For this review, take the finished solid that the model builds, in its own axes (mm). A direction names the side the tool comes from. Give positions to 0.01 mm unless a question says otherwise; leave off trailing zeros. Write each loop counter-clockwise with the first axis right and the second up, starting at its lowest first coordinate (ties: lowest second). Pieces come first, ordered by that corner, then holes. Notation, with made-up numbers: (76.5, -34) -> (108.5, -34) arc R17 cw to (108.5, -23) -> close; hole circle Ø7 at (13, -30.75). An arc over 180 degrees is marked (long way). Return JSON: item names as keys, results as strings.
from build123d import *

# Parameters (mm, degrees)
PAD_DEPTH    = 10
SKETCH001_R  = 2
POCKET_DEPTH = 31
CHAMFER_SIZE = 4
FILLET_R     = 4


with BuildPart() as part:
    # Sketch → Pad (new body)
    with BuildSketch(Plane.XY):
        Polygon((-9, 7.5), (9, 7.5), (9, 22), (14, 22), (14, -22), (9, -22), (9, -7.5), (-9, -7.5), (-9, -22), (-14, -22), (-14, 22), (-9, 22), align=None)
    extrude(amount=PAD_DEPTH)

    # Sketch001 (on Face4 of Pad) → Pocket (cut)
    with BuildSketch(Plane.YZ.offset(14)):
        with Locations((-17, 5)):
            Circle(SKETCH001_R)
        with Locations((17, 5)):
            Circle(SKETCH001_R)
    extrude(amount=-POCKET_DEPTH, mode=Mode.SUBTRACT)

    # Chamfer
    chamfer_edges = [part.edges().sort_by_distance(p)[0] for p in [
        (0, 7.5, 10),
        (0, -7.5, 10),
        (0, 7.5, 0),
        (0, -7.5, 0),
    ]]
    chamfer(chamfer_edges, length=CHAMFER_SIZE)

    # Fillet
    fillet_edges = [part.edges().sort_by_distance(p)[0] for p in [
        (11.5, 22, 0),
        (-11.5, 22, 0),
        (11.5, 22, 10),
        (-11.5, 22, 10),
        (11.5, -22, 10),
        (-11.5, -22, 10),
        (-11.5, -22, 0),
        (11.5, -22, 0),
    ]]
    fillet(fillet_edges, radius=FILLET_R)


solid = part.part
1. For faces 1 (the flat face through (-0.1, 5.5, 8)), 2 (the cylindrical face through (11.535, 20.797, 1.141)), 3 (the flat face through (-0.1, 5.5, 2)), list the 3-axis set-ups (+Z, -Z, +X, -X, +Y, -Y) from which the entire face can be reached by the end or side of a thin tool; tool diameter is ignored.
Results found:
{"face 1": "+Z, +Y", "face 2": "-Z, +X, -X, +Y", "face 3": "-Z, +Y"}
2. Add section C-C, the plane y = 10. State the section outline as (x, z) points.
Results found:
{"outline": "(-14, 0) -> (-9, 0) -> (-9, 10) -> (-14, 10) -> close; (9, 0) -> (14, 0) -> (14, 10) -> (9, 10) -> close"}
3. For pin 1 (1 mm diameter, centred on x = -3, z = 4.5, fed in from +Y); pin 2 (2 mm diameter, centred on x = -0.5, z = 5, fed in from -Y), all flat-tipped, find the tip position at first contact; note any pin that passes through.
Results found:
{"pin 1": "stops at y = 7.5", "pin 2": "stops at y = -7.5"}
4. To check wall thickness, follow probe 1 along Z at (x, y) = (-10.9, 17); probe 2 along X at (y, z) = (10, 8.25); probe 3 along Y at (x, z) = (6.75, 5.5). State the ranges of each line that lie inside material, in increasing order.
Results found:
{"probe 1": "z = 0 to 3, 7 to 10", "probe 2": "x = -14 to -9, 9 to 14", "probe 3": "y = -7.5 to 7.5"}
5. The part is to be moulded in two halves that separate along Y. For faces 4 (the cylindrical face through (-11, -19, 5)), 5 (the flat face through (0, 7.5, 5)), 6 (the flat face through (12, -22, 5)), say which applies: +Y half, -Y half, draft (parallel to the pull), parting line (faces both ways), or undercut.
Results found:
{"face 4": "undercut", "face 5": "+Y half", "face 6": "-Y half"}
6. Add section B-B, the plane z = 5. State the section outline as (x, y) points, plus the area to 3 significant figures.
Results found:
{"outline": "(-14, -22) -> (-9, -22) -> (-9, -19) -> (-14, -19) -> close; (-14, -15) -> (-9, -15) -> (-9, -7.5) -> (9, -7.5) -> (9, -15) -> (14, -15) -> (14, 15) -> (9, 15) -> (9, 7.5) -> (-9, 7.5) -> (-9, 15) -> (-14, 15) -> close; (-14, 19) -> (-9, 19) -> (-9, 22) -> (-14, 22) -> close; (9, -22) -> (14, -22) -> (14, -19) -> (9, -19) -> close; (9, 19) -> (14, 19) -> (14, 22) -> (9, 22) -> close", "area": "630 mm²"}
7. Add section D-D, the plane y = -5. State the section outline as (x, z) points, plus the area to 3 significant figures.
Results found:
{"outline": "(-14, 0) -> (-9, 0) -> (-9, 1.5) -> (9, 1.5) -> (9, 0) -> (14, 0) -> (14, 10) -> (9, 10) -> (9, 8.5) -> (-9, 8.5) -> (-9, 10) -> (-14, 10) -> close", "area": "226 mm²"}
8. Add section A-A, the plane y = 17. State the section outline as (x, z) points.
Results found:
{"outline": "(-14, 0) -> (-9, 0) -> (-9, 3) -> (-14, 3) -> close; (-14, 7) -> (-9, 7) -> (-9, 10) -> (-14, 10) -> close; (9, 0) -> (14, 0) -> (14, 3) -> (9, 3) -> close; (9, 7) -> (14, 7) -> (14, 10) -> (9, 10) -> close"}
